Build history of the part. All positions in model axes, mm. A direction names the side the tool comes from. Coordinates: 2 decimals unless noted, no trailing zeros. Write each loop counter-clockwise with the first axis right and the second up, starting at its lowest first coordinate (ties: lowest second). Pieces come first, ordered by that corner, then holes. Notation, with made-up numbers: (37, 43.5) -> (90, 43.5) arc R22 cw to (90, 67.5) -> close; hole circle Ø10 at (50.5, 21.25). An arc over 180 degrees is marked (long way). Write each question's results on one line, items separated by ' | '. Start each with the question number.
Q1. Drop flat-ended pins along their axis: pin 1 Ø6 at (x, y) = (-6, 3) entering from +Z; pin 2 Ø2.5 at (y, z) = (-6, 7.5) entering from +X; pin 3 Ø1.8 at (x, z) = (2, 7) entering from -Y. Give the stop position or say it passes through.
Q2. Saw through at A-A on x = 0. Give the cut face in (y, z).
Q3. Two-plate mould, pull along Y, no slides. Class faces 6 (the face through (0, -2, 2)), 7 (the face through (-8.99, -5.95, 8.2)), 8 (the face through (0, -3, 7)), 9 (the face through (-15, 0, 2)): released by +Y, released by -Y, zero draft, split by the parting line, or undercut.
Q4. Tool access for faces 1 (the face through (-10, -7.4, 7)), 2 (the face through (1.13, -5.93, 8.5)), 3 (the face through (10, -7.4, 5.6)), 4 (the face through (0, -6, 10)), 5 (the face through (0, -9, 7)): list every direction of +Z, -Z, +X, -X, +Y, -Y with a clear straight run to the whole face (end or side of a thin tool).
Q5. Saw through at D-D on x = 7.75. Give the cut face in (y, z).
Q6. Saw through at C-C on y = -6. Give the cut face in (x, z).
Q7. Drill centre lines: line 1 (Y direction, x = 0, z = 1); line 2 (Y direction, x = -2.5, z = 7); line 3 (Z direction, x = 14, y = -5.75). Where is each one in solid material? Low to high.
Q8. Saw through at B-B on z = 7. Give the cut face in (x, y).
from build123d import *

# Parameters (mm, degrees)
SKETCH1_W           = 30
SKETCH1_H           = 20
SKETCH1_R           = 2
BOSS_EXTRUDE1_DEPTH = 4
SKETCH2_W           = 20
SKETCH2_H           = 6
BOSS_EXTRUDE2_DEPTH = 6
SKETCH4_R           = 1.5
CUT_EXTRUDE1_DEPTH  = 18
SKETCH5_R           = 1.2
CUT_EXTRUDE2_DEPTH  = 6


with BuildPart() as part:
    # Sketch1 → Boss-Extrude1 (new body)
    with BuildSketch(Plane.XY):
        Rectangle(SKETCH1_W, SKETCH1_H)
        Circle(SKETCH1_R, mode=Mode.SUBTRACT)
    extrude(amount=BOSS_EXTRUDE1_DEPTH)

    # Sketch2 → Boss-Extrude2 (add)
    with BuildSketch(Plane.XY.offset(4)):
        with Locations((0, -6)):
            Rectangle(SKETCH2_W, SKETCH2_H)
    extrude(amount=BOSS_EXTRUDE2_DEPTH)

    # Sketch4 → Cut-Extrude1 (cut)
    with BuildSketch(Plane(origin=(10, 0, 0), x_dir=(0, 0, -1), z_dir=(1, 0, 0))):
        with Locations((-7, -6)):
            Circle(SKETCH4_R)
    extrude(amount=-CUT_EXTRUDE1_DEPTH, mode=Mode.SUBTRACT)

    # Sketch5 → Cut-Extrude2 (cut)
    with BuildSketch(Plane(origin=(-8, 0, 0), x_dir=(0, 0, -1), z_dir=(1, 0, 0))):
        with Locations((-7, -6)):
            Circle(SKETCH5_R)
    extrude(amount=-CUT_EXTRUDE2_DEPTH, mode=Mode.SUBTRACT)


solid = part.part
Returned:
1) pin 1: stops at z = 4 | pin 2: stops at x = 10 | pin 3: stops at y = -9
2) outline: (-10, 0) -> (-2, 0) -> (-2, 4) -> (-3, 4) -> (-3, 10) -> (-9, 10) -> (-9, 4) -> (-10, 4) -> close; (2, 0) -> (10, 0) -> (10, 4) -> (2, 4) -> close; hole circle Ø3 at (-6, 7)
3) face 6: undercut | face 7: undercut | face 8: released by +Y | face 9: zero draft
4) face 1: +Z, -X, +Y, -Y | face 2: +X | face 3: +Z, +X, +Y, -Y | face 4: +Z, +X, -X, +Y, -Y | face 5: +Z, +X, -X, -Y
5) outline: (-10, 0) -> (10, 0) -> (10, 4) -> (-3, 4) -> (-3, 10) -> (-9, 10) -> (-9, 4) -> (-10, 4) -> close; hole circle Ø3 at (-6, 7)
6) outline: (-15, 0) -> (15, 0) -> (15, 4) -> (10, 4) -> (10, 5.5) -> (-8, 5.5) -> (-8, 5.8) -> (-10, 5.8) -> (-10, 4) -> (-15, 4) -> close; (-10, 8.2) -> (-8, 8.2) -> (-8, 8.5) -> (10, 8.5) -> (10, 10) -> (-10, 10) -> close
7) line 1: y = -10 to -2, 2 to 10 | line 2: y = -9 to -7.5, -4.5 to -3 | line 3: z = 0 to 4
8) outline: (-10, -9) -> (10, -9) -> (10, -7.5) -> (-8, -7.5) -> (-8, -7.2) -> (-10, -7.2) -> close; (-10, -4.8) -> (-8, -4.8) -> (-8, -4.5) -> (10, -4.5) -> (10, -3) -> (-10, -3) -> close
